from build123d import *

# Parameters (mm, degrees)
BOSS_EXTRUDE2_DEPTH              = 12
BOSS_EXTRUDE3_DEPTH              = 2
CUT_EXTRUDE1_DEPTH               = 3
FILLET1_R                        = 3
TAP_DRILL_FOR_M10X1_5_TAP1_D     = 8.5
TAP_DRILL_FOR_M10X1_5_TAP1_DEPTH = 12.55
TAP_DRILL_FOR_M10X1_5_TAP1_TIP   = 4.25


with BuildPart() as part:
    # Sketch2 → Boss-Extrude2 (new body)
    with BuildSketch(Plane(origin=(0, 0, 0), x_dir=(1, 0, 0), z_dir=(0, 1, 0))):
        with BuildLine():
            Line((12, 0), (146, 0))
            ThreePointArc((146, 0), (154.485281374, 3.514718626), (158, 12))
            Line((158, 12), (158, 62))
            ThreePointArc((158, 62), (154.485281374, 70.485281374), (146, 74))
            Line((146, 74), (12, 74))
            ThreePointArc((12, 74), (3.514718626, 70.485281374), (0, 62))
            Line((0, 62), (0, 12))
            ThreePointArc((0, 12), (3.514718626, 3.514718626), (12, 0))
        make_face()
    extrude(amount=BOSS_EXTRUDE2_DEPTH)

    # 3DSketch2 → Boss-Extrude3 (add)
    with BuildSketch(Plane(origin=(112, 12, 0), x_dir=(-0.6656148469584017, 0, -0.7462954344685109), z_dir=(0, -1, 0))):
        Polygon((0, 0), (55.225862151, 49.255498675), (99.15644205, 0), (43.930579899, -49.255498675), align=None)
    extrude(amount=-BOSS_EXTRUDE3_DEPTH)

    # 3DSketch3 → Cut-Extrude1 (cut)
    with BuildSketch(Plane(origin=(104, 0, -74), x_dir=(-0.5598574112779868, 0, 0.8285889686914202), z_dir=(0, -1, 0))):
        Polygon((0, 0), (61.315583683, -41.429448435), (89.308454247, 0), (27.992870564, 41.429448435), align=None)
    extrude(amount=-CUT_EXTRUDE1_DEPTH, mode=Mode.SUBTRACT)

    # Fillet1
    fillet1_edges = [part.edges().sort_by_distance(p)[0] for p in [
        (104, 3, -37),
        (54, 3, -37),
    ]]
    fillet(fillet1_edges, radius=FILLET1_R - 0.0001)  # a hair under: the kernel refuses the full size

    # Tap Drill for M10x1.5 Tap1
    with Locations(Plane(origin=(0, 12, 0), x_dir=(1, 0, 0), z_dir=(0, 1, 0))):
        with Locations((146, 12), (146, 62), (12, 12), (12, 62)):
            Hole(TAP_DRILL_FOR_M10X1_5_TAP1_D / 2, depth=TAP_DRILL_FOR_M10X1_5_TAP1_DEPTH)
            with Locations((0, 0, -(TAP_DRILL_FOR_M10X1_5_TAP1_DEPTH + TAP_DRILL_FOR_M10X1_5_TAP1_TIP / 2))):  # 90° drill point
                Cone(0, TAP_DRILL_FOR_M10X1_5_TAP1_D / 2, TAP_DRILL_FOR_M10X1_5_TAP1_TIP, mode=Mode.SUBTRACT)


solid = part.part
Read the model definition and answer for the solid it produces. Units are mm, in the model's axes. A direction names the side the tool comes from. Give positions to 0.01 mm unless a question says otherwise; leave off trailing zeros. Write each loop counter-clockwise with the first axis right and the second up, starting at its lowest first coordinate (ties: lowest second). Pieces come first, ordered by that corner, then holes. Notation, with made-up numbers: (-36.5, 15.5) -> (9.5, 15.5) arc R35 ccw to (9.5, 53.5) -> close; hole circle Ø9 at (77.5, 85). An arc over 180 degrees is marked (long way). Answer as a JSON object with one key per item and string values. Group by question number.
1) The mould has two halves that part along X. Classify faces 1 (the cylindrical face through (154.58, 5.92, -70.39)), 2 (the cylindrical face through (3.61, 5.92, -70.58)), 3 (the flat face through (135, 12, -38)), 4 (the cylindrical face through (54.86, 2.1, -37.52)): +X half, -X half, draft (parallel to the pull), parting line (faces both ways), or undercut.
2) Each of these flat-tipped pins is pushed along its axis until it touches: P1, Ø1, axis at x = 33, z = -14.5, coming from the +Y side; P2, Ø2, axis at y = 13.5, z = -38, coming from the -X side; P3, Ø13.5, axis at x = 12, z = -62, coming from the -Y side; P4, Ø7.5, axis at x = 146, z = -62, coming from the -Y side. Where does it stop, or does it pass through?
3) A tool of negligible diameter and unlimited length cuts with its end or side. For faces 5 (the flat face through (131, 0, -38)), 6 (the cylindrical face through (103.1, 2.14, -36.48)), 7 (the flat face through (23, 12, -38)), from which of +Z, -Z, +X, -X, +Y, -Y can it reach the whole face along a straight path? Write none if from no direction.
4) Find section C-C (x = 61). Write down the section's boundary in (y, z).
5) Find section B-B (y = 1.5). Write down the section's boundary in (x, z).
6) Find section A-A (y = 9.75). Write down the section's boundary in (x, z), and give its area (3 significant figures).
7) Consider L1, parallel to Z at x = 146, y = 5; L2, parallel to X at y = 7, z = -62; L3, parallel to Y at x = 27.5, z = -44.5. Determine where each line is inside the solid, lowest interval first. Write a range as from..to.
Values follow:
{
 "1": {"face 1": "+X half", "face 2": "-X half", "face 3": "draft", "face 4": "undercut"},
 "2": {"P1": "stops at y = 12", "P2": "stops at x = 46", "P3": "stops at y = 0", "P4": "passes through"},
 "3": {"face 5": "+Z, -Z, +X, -X, -Y", "face 6": "+Z, -Z, -Y", "face 7": "+Z, -Z, -X, +Y"},
 "4": {"outline": "(3, -74) -> (14, -74) -> (14, 0) -> (3, 0) -> close"},
 "5": {"outline": "(0, -62) arc R12 ccw to (12, -74) -> (54.4, -74) -> (54.4, 0) -> (12, 0) arc R12 ccw to (0, -12) -> close; (103.6, -74) -> (146, -74) arc R12 ccw to (158, -62) -> (158, -12) arc R12 ccw to (146, 0) -> (103.6, 0) -> close; hole circle Ø8.5 at (12, -62); hole circle Ø8.5 at (12, -12); hole circle Ø8.5 at (146, -62); hole circle Ø8.5 at (146, -12)"},
 "6": {"outline": "(0, -62) arc R12 ccw to (12, -74) -> (146, -74) arc R12 ccw to (158, -62) -> (158, -12) arc R12 ccw to (146, 0) -> (12, 0) arc R12 ccw to (0, -12) -> close; hole circle Ø8.5 at (12, -62); hole circle Ø8.5 at (12, -12); hole circle Ø8.5 at (146, -62); hole circle Ø8.5 at (146, -12)", "area": "11,300 mm2"},
 "7": {"L1": "z = -74..-66.25, -57.75..-16.25, -7.75..0", "L2": "x = 0..7.75, 16.25..141.75, 150.25..158", "L3": "y = 0..12"}
}
